Can you work these out from the drawing? Everything is in mm from the part's minimum corner. A direction names the side the tool comes from. Give positions to 0.01 mm unless a question says otherwise; leave off trailing zeros. Order: outer loops, then holes, each group sorted by start corner. A loop starts at its lowest first (then second) coordinate and runs counter-clockwise, first axis right, second up. Notation, with made-up numbers: (80, 20) - (95, 20) arc R8 ccw to (95, 32) - close; hole circle Ø8 at (5, 19.25). An arc over 180 degrees is marked (long way). Answer as a JSON object with one key per item and string values.
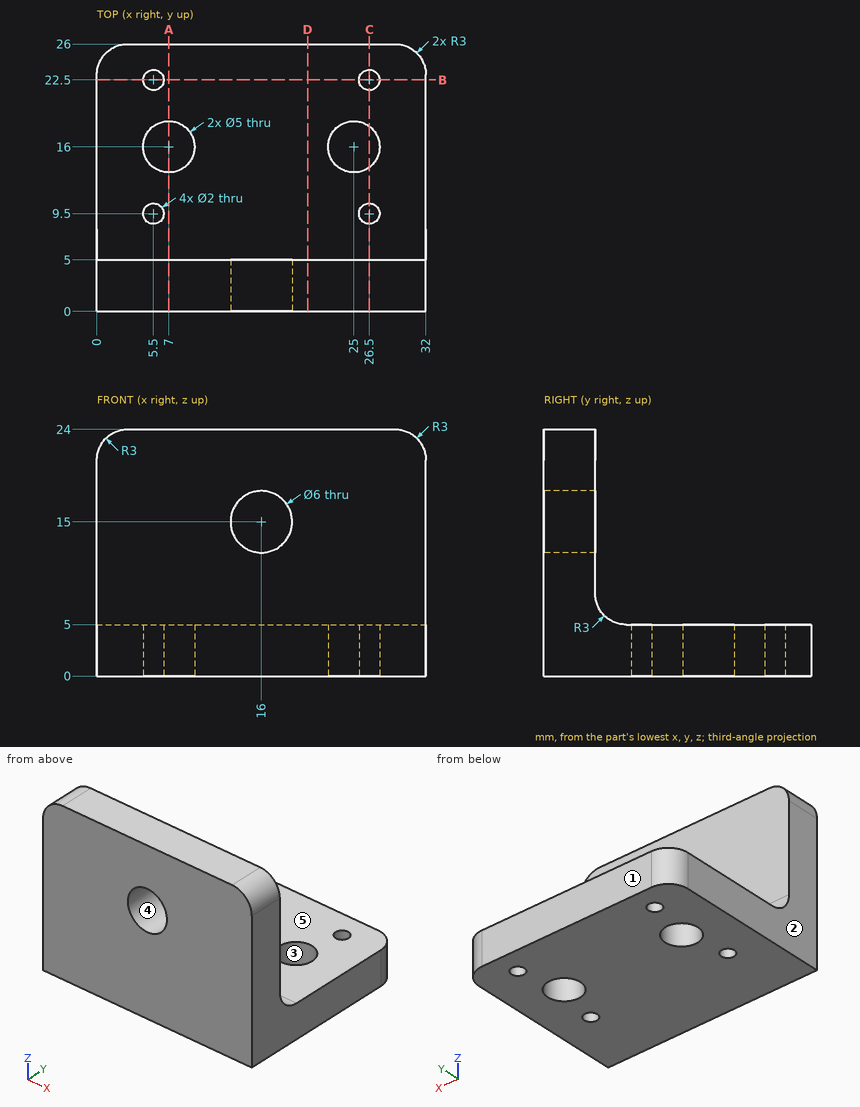
Q1. I need wall thicknesses on L1, parallel to Y at x = 5.5, z = 1.9; L2, parallel to Z at x = 16, y = 3.45; L3, parallel to Y at x = 7, z = 2.05. Which ranges of each line are inside material? Lowest first, please.
Recorded:
{"L1": "y = 0 to 8.5, 10.5 to 14, 18 to 21.5, 23.5 to 26", "L2": "z = 0 to 12, 18 to 24", "L3": "y = 0 to 13.5, 18.5 to 26"}
Q2. If we section it at B-B, the plane y = 22.5: Please give me the cut outline in (x, z).
Recorded:
{"outline": "(0, 0) - (4.5, 0) - (4.5, 5) - (0, 5) - close; (6.5, 0) - (25.5, 0) - (25.5, 5) - (6.5, 5) - close; (27.5, 0) - (32, 0) - (32, 5) - (27.5, 5) - close"}
Q3. We'd pull the mould along Y, two halves only. Please class the marked faces 1, 2 and 3: released by +Y, released by -Y, zero draft, split by the parting line, or undercut.
Recorded:
{"face 1": "released by +Y", "face 2": "zero draft", "face 3": "undercut"}
Q4. If we section it at D-D, the plane x = 20.5: Please give me the cut outline in (y, z).
Recorded:
{"outline": "(0, 0) - (26, 0) - (26, 5) - (8, 5) arc R3 cw to (5, 8) - (5, 24) - (0, 24) - close"}
Q5. If we section it at C-C, the plane x = 26.5: Please give me the cut outline in (y, z).
Recorded:
{"outline": "(0, 0) - (8.5, 0) - (8.5, 5) - (8, 5) arc R3 cw to (5, 8) - (5, 24) - (0, 24) - close; (10.5, 0) - (14, 0) - (14, 5) - (10.5, 5) - close; (18, 0) - (21.5, 0) - (21.5, 5) - (18, 5) - close; (23.5, 0) - (26, 0) - (26, 5) - (23.5, 5) - close"}
Q6. If we section it at A-A, the plane x = 7: Please give me the cut outline in (y, z), then the cut area to 3 significant figures.
Recorded:
{"outline": "(0, 0) - (13.5, 0) - (13.5, 5) - (8, 5) arc R3 cw to (5, 8) - (5, 24) - (0, 24) - close; (18.5, 0) - (26, 0) - (26, 5) - (18.5, 5) - close", "area": "202 mm^2"}
Q7. I'm going to push flat-ended pins straight in: pin 1 Ø6 at (x, y) = (25, 16) entering from +Z; pin 2 Ø1.8 at (x, y) = (26.5, 22.5) entering from +Z; pin 3 Ø9.5 at (x, z) = (16, 15) entering from +Y; pin 4 Ø10 at (x, y) = (9.5, 12) entering from +Z. Where does each tip first touch, or does it pass through?
Recorded:
{"pin 1": "stops at z = 5", "pin 2": "passes through", "pin 3": "stops at y = 5", "pin 4": "stops at z = 5.17"}
Q8. Which directions (+Z, -Z, +X, -X, +Y, -Y) give clear straight access to the entire face, cutting with the end or side of a thin tool? Please do the marked faces 4 and 5.
Recorded:
{"face 4": "+Y, -Y", "face 5": "+Z, +X, -X, +Y"}
